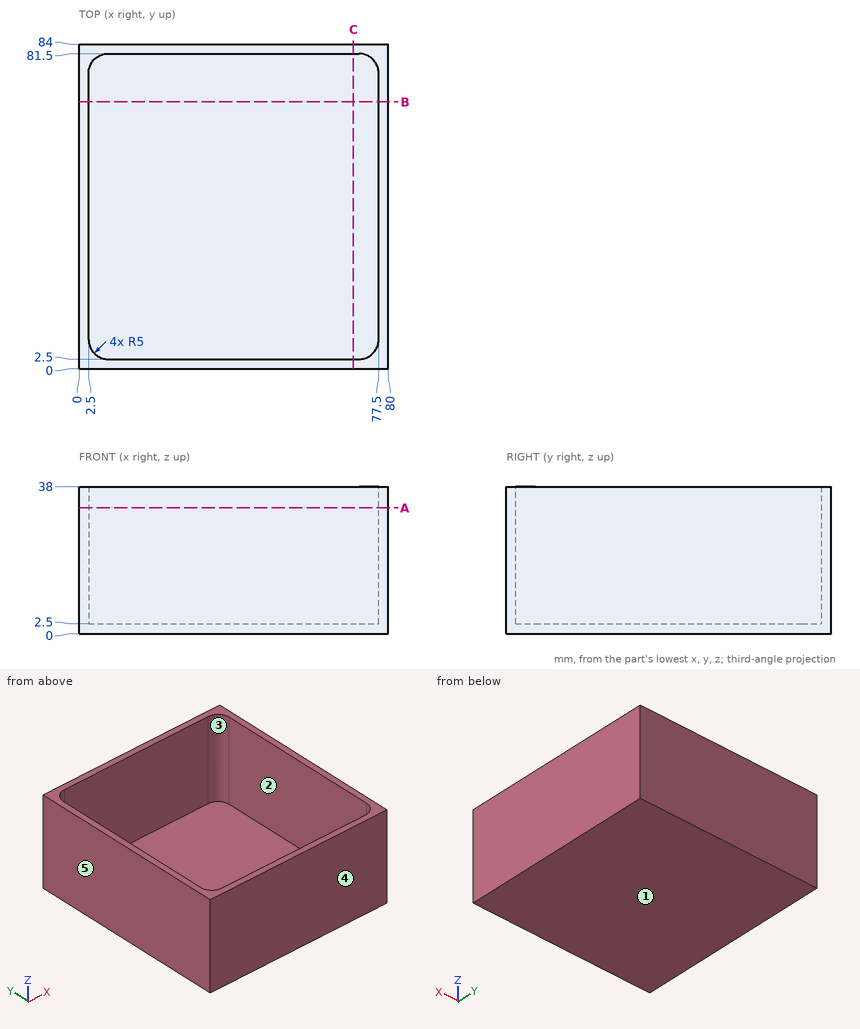
Design review of the part shown in the three views and the two pictorial views. Dimensions are in mm from the part's minimum x, y and z. A direction names the side the tool comes from. Give positions to 0.01 mm unless a question says otherwise; leave off trailing zeros. Loops run counter-clockwise (first coordinate to the right, second up) from the corner with the lowest first, then second, coordinate; pieces in that order, holes last. Notation, with made-up numbers: M 38,88.25 L 51,88.25 A23 ccw 51,119.25 Z; hole C 83.25,7.25 d11. An arc over 180 degrees is marked long. Put each result on its own line as item: value. Start each with the question number.
(1) Wall thickness on L1, parallel to X at y = 29.5, z = 35; L2, parallel to Y at x = 66.5, z = 28; L3, parallel to Z at x = 51.5, y = 21: over which ranges is each line inside the solid? List them lowest first.
(2) Add section A-A, the plane z = 32.5. Write out the cut boundary in (x, y), then the cut area to 3 significant figures.
(3) The part is to be moulded in two halves that separate along X. For the marked faces 3, 4 and 5, say which applies: +X half, -X half, draft (parallel to the pull), parting line (faces both ways), or undercut.
(4) Machinability: for the marked faces 1 and 2, which of the approach directions +Z, -Z, +X, -X, +Y, -Y give a long, thin tool a straight path to every point of the face, cutting with its end or side? Answer none if there is none.
(5) Add section C-C, the plane x = 71. Write out the cut boundary in (y, z), then the cut area to 4 significant figures.
(6) Add section B-B, the plane y = 69. Write out the cut boundary in (x, z).
(7) For pin 1 (10.5 mm diameter, centred on x = 31.5, z = 12.5, fed in from -Y); pin 2 (1.5 mm diameter, centred on x = 13.5, y = 28.5, fed in from +Z), all flat-tipped, find the tip position at first contact; note any pin that passes through.
Result:
1. L1: x = 0 to 2.5, 77.5 to 80
1. L2: y = 0 to 2.5, 81.5 to 84
1. L3: z = 0 to 2.5
2. outline: M 0,0 L 80,0 L 80,84 L 0,84 Z; hole M 2.5,7.5 A5 ccw 7.5,2.5 L 72.5,2.5 A5 ccw 77.5,7.5 L 77.5,76.5 A5 ccw 72.5,81.5 L 7.5,81.5 A5 ccw 2.5,76.5 Z
2. area: 816 mm^2
3. face 3: undercut
3. face 4: draft
3. face 5: -X half
4. face 1: -Z, +X, -X, +Y, -Y
4. face 2: +Z
5. outline: M 0,0 L 84,0 L 84,38 L 81.5,38 L 81.5,2.5 L 2.5,2.5 L 2.5,38 L 0,38 Z
5. area: 387.5 mm^2
6. outline: M 0,0 L 80,0 L 80,38 L 77.5,38 L 77.5,2.5 L 2.5,2.5 L 2.5,38 L 0,38 Z
7. pin 1: stops at y = 0
7. pin 2: stops at z = 2.5
